Work out the finished part from the listing and answer in its coordinate system (mm). Face numbers are marked on the shaded views. A direction names the side the tool comes from. Coordinates: 2 decimals unless noted, no trailing zeros. Loops run counter-clockwise (first coordinate to the right, second up) from the corner with the lowest first, then second, coordinate; pieces in that order, holes last. Notation, with made-up numbers: M 76.25,66 L 98.25,66 A17 cw 98.25,98 Z; hole C 47,59 d10. An arc over 180 degrees is marked long. Write each question's results on one line, items separated by ' | '.
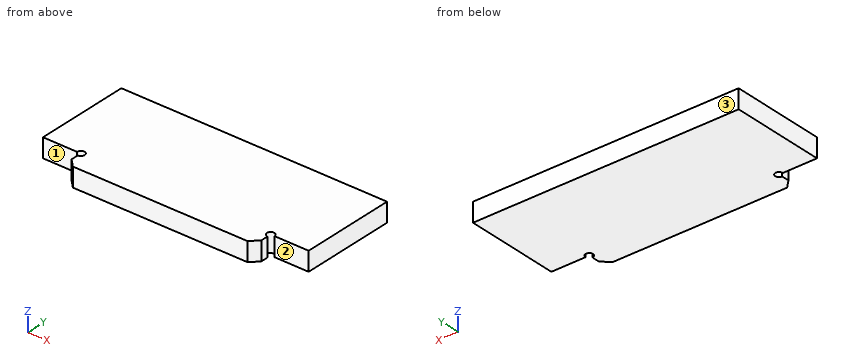
```python
from build123d import *

# Parameters (mm, degrees)
EXTRUDE_1_DEPTH = 2.5


with BuildPart() as part:
    # 草圖1 → 填料-伸長1 (new, symmetric)
    with BuildSketch(Plane.XY):
        with BuildLine():
            Line((-25, 2), (-23, 0))
            Line((-23, 0), (23, 0))
            Line((23, 0), (25, 2))
            Line((25, 2), (25, 4))
            ThreePointArc((25, 4), (24.292893219, 5.707106781), (26, 5))
            Line((26, 5), (35, 5))
            Line((35, 5), (35, 30))
            Line((35, 30), (-35, 30))
            Line((-35, 30), (-35, 5))
            Line((-35, 5), (-26, 5))
            ThreePointArc((-26, 5), (-24.292893219, 5.707106781), (-25, 4))
            Line((-25, 4), (-25, 2))
        make_face()
    extrude(amount=EXTRUDE_1_DEPTH, both=True)


solid = part.part
```
1) Find section B-B, the plane x = -29.5. Give the vertices of the cut face in (y, z).
Check result:
outline: M 5,-2.5 L 30,-2.5 L 30,2.5 L 5,2.5 Z
2) Given pin 1 Ø1.6 at (y, z) = (2.5, 1) entering from -X; pin 2 Ø1.5 at (x, z) = (-30, 0.5) entering from -Y; pin 3 Ø2 at (y, z) = (3.5, -1) entering from +X, each flat-ended and moving along its own axis, determine where each tip first touches the part or whether it passes through.
Check result:
pin 1: x = -25 | pin 2: y = 5 | pin 3: x = 25
3) Which of the six approach directions +Z, -Z, +X, -X, +Y, -Y give full straight-line access (tool end or side, diameter ignored) to the marked faces 1, 2 and 3?
Check result:
face 1: +Z, -Z, -X, -Y | face 2: +Z, -Z, +X, -Y | face 3: +Z, -Z, +X, -X, +Y
4) A straight line is drawn through the part: probe 1 along Y at (x, z) = (31.5, -0.55). Find the intervals that lie inside material, in ascending order. Write a range as [from, to].
Check result:
probe 1: [5, 30]
5) Find section A-A, the plane z = 0.2. Give the vertices of the cut face in (x, y), and give its area (3 significant figures).
Check result:
outline: M -35,5 L -26,5 A1 cw long -25,4 L -25,2 L -23,0 L 23,0 L 25,2 L 25,4 A1 cw long 26,5 L 35,5 L 35,30 L -35,30 Z | area: 1,990 mm^2
6) Find section C-C, the plane y = 3. Give the vertices of the cut face in (x, z).
Check result:
outline: M -25,-2.5 L 25,-2.5 L 25,2.5 L -25,2.5 Z
